Design review of the part built by this model. Coordinates are the model's own, in mm. A direction names the side the tool comes from. Give positions to 0.01 mm unless a question says otherwise; leave off trailing zeros. Order: outer loops, then holes, each group sorted by start corner. A loop starts at its lowest first (then second) coordinate and runs counter-clockwise, first axis right, second up.
```python
from build123d import *

# Parameters (mm, degrees)
BOSS_EXTRUDE1_DEPTH = 0.7112
SKETCH2_R           = 2.0955
CUT_EXTRUDE1_DEPTH  = 2.4224
CUT_EXTRUDE2_DEPTH  = 49.6824
SKETCH4_W           = 0.6477
SKETCH4_H           = 7.286325031
CUT_EXTRUDE4_DEPTH  = 25.4


with BuildPart() as part:
    # Sketch1 → Boss-Extrude1 (new body, symmetric)
    with BuildSketch(Plane.XY):
        with BuildLine():
            Line((54.87519109, 58.900672801), (54.87519109, 25.880672801))
            Line((54.87519109, 25.880672801), (60.323650659, 17.097007032))
            ThreePointArc((60.323650659, 17.097007032), (61.02184914, 16.738358549), (61.666295368, 17.186464467))
            ThreePointArc((61.666295368, 17.186464467), (64.337974251, 25.783780398), (64.874140477, 34.770672801))
            Line((64.874140477, 34.770672801), (63.892088906, 50.780757429))
            ThreePointArc((63.892088906, 50.780757429), (63.598614861, 52.297421008), (64.78119109, 53.291357066))
            Line((64.78119109, 53.291357066), (64.78119109, 62.189940891))
            ThreePointArc((64.78119109, 62.189940891), (60.720306841, 64.227784091), (56.90719109, 61.757210459))
            Line((56.90719109, 61.757210459), (56.90719109, 59.662672801))
            ThreePointArc((56.90719109, 59.662672801), (56.684006458, 59.123857434), (56.14519109, 58.900672801))
            Line((56.14519109, 58.900672801), (54.87519109, 58.900672801))
        make_face()
    extrude(amount=BOSS_EXTRUDE1_DEPTH, both=True)

    # Sketch2 → Cut-Extrude1 (cut, through all)
    with BuildSketch(Plane.XY.offset(0.7112)):
        with Locations((60.97119109, 59.662672801)):
            Circle(SKETCH2_R)
    extrude(amount=-CUT_EXTRUDE1_DEPTH, mode=Mode.SUBTRACT)

    # Sketch3 → Cut-Extrude2 (cut)
    with BuildSketch(Plane(origin=(0, 0, 0), x_dir=(1, 0, 0), z_dir=(0, 1, 0))):
        Polygon((64.78119109, 0.0635), (54.87519109, 0.7112), (64.78119109, 0.7112), align=None)
        Polygon((54.87519109, -0.7112), (64.78119109, -0.0635), (64.78119109, -0.7112), align=None)
    extrude(amount=CUT_EXTRUDE2_DEPTH, mode=Mode.SUBTRACT)

    # Sketch4 → Cut-Extrude4 (cut)
    with BuildSketch(Plane.ZY.offset(-64.78119109)):
        with Locations((0.38735, 32.642835537)):
            Rectangle(SKETCH4_W, SKETCH4_H)
        with Locations((-0.38735, 32.642835537)):
            Rectangle(SKETCH4_W, SKETCH4_H)
    extrude(amount=-CUT_EXTRUDE4_DEPTH, mode=Mode.SUBTRACT)


solid = part.part
```
1. Take a section at B-B (y = 56.5). State the section outline as (x, z) points.
Recorded:
outline: (54.88, -0.71) - (64.78, -0.71) - (64.78, 0.71) - (54.88, 0.71) - close
2. Take a section at C-C (x = 58). State the section outline as (y, z) points.
Recorded:
outline: (20.84, -0.51) - (49.68, -0.51) - (49.68, -0.71) - (63.14, -0.71) - (63.14, 0.71) - (49.68, 0.71) - (49.68, 0.51) - (20.84, 0.51) - close
3. For pin 1 (0.6 mm diameter, centred on x = 55.5, z = 0, fed in from +Y); pin 2 (4 mm diameter, centred on x = 64, y = 25.5, fed in from -Z); pin 3 (4 mm diameter, centred on x = 60.97, y = 59.66, fed in from -Z); pin 4 (0.7 mm diameter, centred on x = 59, z = 0.5, fed in from -Y), all flat-tipped, find the tip position at first contact; note any pin that passes through.
Recorded:
pin 1: stops at y = 58.9
pin 2: stops at z = -0.25
pin 3: passes through
pin 4: stops at y = 18.68
4. Take a section at A-A (x = 61). State the section outline as (y, z) points.
Recorded:
outline: (16.74, -0.31) - (49.68, -0.31) - (49.68, -0.71) - (57.57, -0.71) - (57.57, 0.71) - (49.68, 0.71) - (49.68, 0.31) - (16.74, 0.31) - close; (61.76, -0.71) - (64.23, -0.71) - (64.23, 0.71) - (61.76, 0.71) - close
5. Take a section at D-D (y = 33.5). State the section outline as (x, z) points, then the cut area to 3 significant figures.
Recorded:
outline: (54.88, -0.71) - (64.78, -0.06) - (64.93, -0.06) - (64.93, 0.06) - (64.78, 0.06) - (54.88, 0.71) - close
area: 7.69 mm2
6. For line 1 along Y through (x, z) = (61, 0.55); line 2 along Y through (x, z) = (61.75, 0.65); line 3 along Z through (x, y) = (59.5, 39.5), list the stretches that pass through material, from the lowest coordinate up.
Recorded:
line 1: y = 49.68 to 57.57, 61.76 to 64.23
line 2: y = 49.68 to 57.72, 61.61 to 64.17
line 3: z = -0.41 to 0.41
7. Machinability: for faces 4 (the face through (59.76, 32.98, 0.39)), 5 (the face through (59.898, 32.979, -0.383)), 6 (the face through (63.6, 52.3, 0)), 7 (the face through (56.907, 61, 0)), which of the approach directions +Z, -Z, +X, -X, +Y, -Y give a long, thin tool a straight path to every point of the face, cutting with its end or side? Answer none if there is none.
Recorded:
face 4: +Z, +X, -Y
face 5: -Z, +X, -Y
face 6: +Z, -Z, +X
face 7: +Z, -Z, -X, +Y
8. Draft analysis for pull direction Y (two halves, no side actions). For faces 1 (the face through (54.875, 43, 0)), 2 (the face through (62.1, 61.43, 0.01)), 3 (the face through (60.79, 64.23, 0.01)), state which applies: pulls with the +Y half, pulls with the -Y half, needs draft (parallel to the pull), parting line crosses it, or undercut.
Recorded:
face 1: needs draft
face 2: undercut
face 3: pulls with the +Y half
